Read the model definition and answer for the solid it produces. Units are mm, in the model's axes. A direction names the side the tool comes from. Round coordinates to 2 decimals unless told otherwise and drop trailing zeros. Order: outer loops, then holes, each group sorted by start corner. A loop starts at its lowest first (then second) coordinate and runs counter-clockwise, first axis right, second up. Notation, with made-up numbers: (-30, -31.75) - (-2, -31.75) arc R15 ccw to (-2, -12.75) - close; hole circle Ø7 at (45, 13.25). An arc over 180 degrees is marked (long way). One line per question, with ' | ' between items. Start each with the question number.
1) For faces 1 (the flat face through (16, 8, 0)), 2 (the flat face through (17.5, -15, 2)), determine the directions among +Z, -Z, +X, -X, +Y, -Y from which every point of the face is accessible in a straight line to the end or side of a thin tool.
2) The part is cut by section A-A, the plane y = -2. Give the vertices of the cut face in (x, z), plus the area to 3 significant figures.
3) The part is cut by section B-B, the plane z = 2.15. Give the vertices of the cut face in (x, y), plus the area to 3 significant figures.
4) Straight lines are drawn through the part: line 1 (X direction, y = -3, z = 2.2); line 2 (X direction, y = 9, z = 2.6); line 3 (Y direction, x = 7.5, z = 4). For each, find the intervals that lie inside material, in ascending order. Write a range as from..to.
5) Flat-ended cylindrical pins translate along their axes: pin 1 (1 mm diameter, centred on x = -5, z = 2.5, fed in from +Y); pin 2 (10 mm diameter, centred on x = 9.5, y = -17.5, fed in from -Z). Find the tip coordinate at first contact, or state that the pin passes through.
6) The part is cut by section D-D, the plane y = 8. Give the vertices of the cut face in (x, z).
7) The mould has two halves that part along X. Classify faces 3 (the flat face through (16, 8, 5)), 4 (the flat face through (-19.5, -15, 2)), 5 (the cylindrical face through (-0.385, 17.496, 2.465)): pulls with the +X half, pulls with the -X half, needs draft (parallel to the pull), parting line crosses it, or undercut.
8) The part is cut by section C-C, the plane x = 0. Give the vertices of the cut face in (y, z), plus the area to 3 significant figures.
Autodesk Inventor part; units mm, degrees
ref_plane "YZ Plane" through (0, 0, 0) normal (1, 0, 0) x (0, 1, 0)
ref_plane "XZ Plane" through (0, 0, 0) normal (0, 1, 0) x (-1, 0, 0)
ref_plane "XY Plane" through (0, 0, 0) normal (0, 0, 1) x (1, 0, 0)
sketch "Sketch1" plane through (0, 0, 0) normal (0, 0, 1) x (1, 0, 0)
  arc A0 (17.5, 0) -> (-17.5, 0) centre (0, 0) ccw
  arc A1 (19.5, 0) -> (-19.5, 0) centre (0, 0) ccw
  line L0 (-19.5, 0) -> (-17.5, 0)
  line L1 (-17.5, 0) -> (-17.5, -10)
  line L2 (-17.5, -10) -> (-19.5, -10)
  line L3 (-19.5, -10) -> (-19.5, 0)
  line L4 (17.5, 0) -> (19.5, 0)
  line L5 (19.5, 0) -> (19.5, -10)
  line L6 (19.5, -10) -> (17.5, -10)
  line L7 (17.5, -10) -> (17.5, 0)
  dimension "d0" = 17.5
  dimension "d1" = 19.5
  dimension "d2" = 10
  dimension "d3" = 10
  dimension "d4" = 2
  dimension "d5" = 2
  dimension "d6" = 19.5
  dimension "d7" = 19.5
extrude "Extrusion1" add sketch "Sketch1" along normal blind 5
sketch "Sketch2" plane through (17.5, -10, 0) normal (0, -1, 0) x (1, 0, 0)
  line L0 (-35, 0) -> (-35, 5)
  line L1 (-37, 5) -> (-35, 5)
  line L2 (-35, 5) -> (-35, 0)
  line L3 (-35, 0) -> (-37, 0)
  line L4 (-37, 0) -> (-37, 5)
  line L5 (2, 0) -> (0, 0)
  line L6 (0, 0) -> (0, 5)
  line L7 (0, 5) -> (2, 5)
  line L8 (2, 5) -> (2, 0)
  point P0 (-17.5, 0)
  dimension "d10" = 2
  dimension "d11" = 5
  dimension "d12" = 2
  dimension "d13" = 5
extrude "Extrusion2" add sketch "Sketch2" along normal blind 20
properties part number "Team29_TubeHolder"
Values:
1) face 1: -Z, +X, -X, +Y, -Y | face 2: +Z, -Z, -Y
2) outline: (-19.5, 0) - (-17.5, 0) - (-17.5, 5) - (-19.5, 5) - close; (17.5, 0) - (19.5, 0) - (19.5, 5) - (17.5, 5) - close | area: 20.0 mm^2
3) outline: (-19.5, -30) - (-17.5, -30) - (-17.5, 0) arc R17.5 cw to (17.5, 0) - (17.5, -30) - (19.5, -30) - (19.5, 0) arc R19.5 ccw to (-19.5, 0) - close | area: 236 mm^2
4) line 1: x = -19.5..-17.5, 17.5..19.5 | line 2: x = -17.3..-15.01, 15.01..17.3 | line 3: y = 15.81..18
5) pin 1: stops at y = 18.97 | pin 2: passes through
6) outline: (-17.78, 0) - (-15.56, 0) - (-15.56, 5) - (-17.78, 5) - close; (15.56, 0) - (17.78, 0) - (17.78, 5) - (15.56, 5) - close
7) face 3: needs draft | face 4: pulls with the -X half | face 5: undercut
8) outline: (17.5, 0) - (19.5, 0) - (19.5, 5) - (17.5, 5) - close | area: 10.0 mm^2
